The figure shows three views and two pictorial views of one solid part (mm, origin at its lowest corner). Answer the questions. A direction names the side the tool comes from. Round coordinates to 2 decimals unless told otherwise and drop trailing zeros. Write each loop counter-clockwise with the first axis right and the second up, starting at its lowest first coordinate (ties: lowest second). Pieces come first, ordered by that corner, then holes. Notation, with made-up numbers: M 15.25,68.5 L 63.25,68.5 A25 cw 63.25,83.5 Z; hole C 5,-36.75 d8. An arc over 180 degrees is marked long. One line per item, written item: value. Start each with the question number.
Q1. Given pin 1 Ø2 at (x, y) = (30.5, 20.5) entering from +Z, flat-ended and moving along its own axis, determine where the tip first touches the part or whether it passes through.
Q2. A tool of negligible diameter and unlimited length cuts with its end or side. For the marked faces 1 and 2, from which of +Z, -Z, +X, -X, +Y, -Y can it reach the whole face along a straight path? Write none if from no direction.
Q3. Find section D-D (x = 30). Write down the section's boundary in (y, z), and give its area (3 significant figures).
Q4. The mould has two halves that part along X. Classify the marked faces 3, 4 and 5: released by +X, released by -X, zero draft, split by the parting line, or undercut.
Q5. Find section C-C (z = 15.5). Write down the section's boundary in (x, y).
Q6. Find section B-B (x = 19). Write down the section's boundary in (y, z), and give its area (3 significant figures).
Q7. Consider probe 1 along Y at (x, z) = (17, 13.5); probe 2 along Y at (x, z) = (4, 14); probe 3 along Y at (x, z) = (15, 13). Determine where each line is inside the solid, lowest interval first.
Q8. Find section A-A (y = 5). Write down the section's boundary in (x, z), and give its area (3 significant figures).
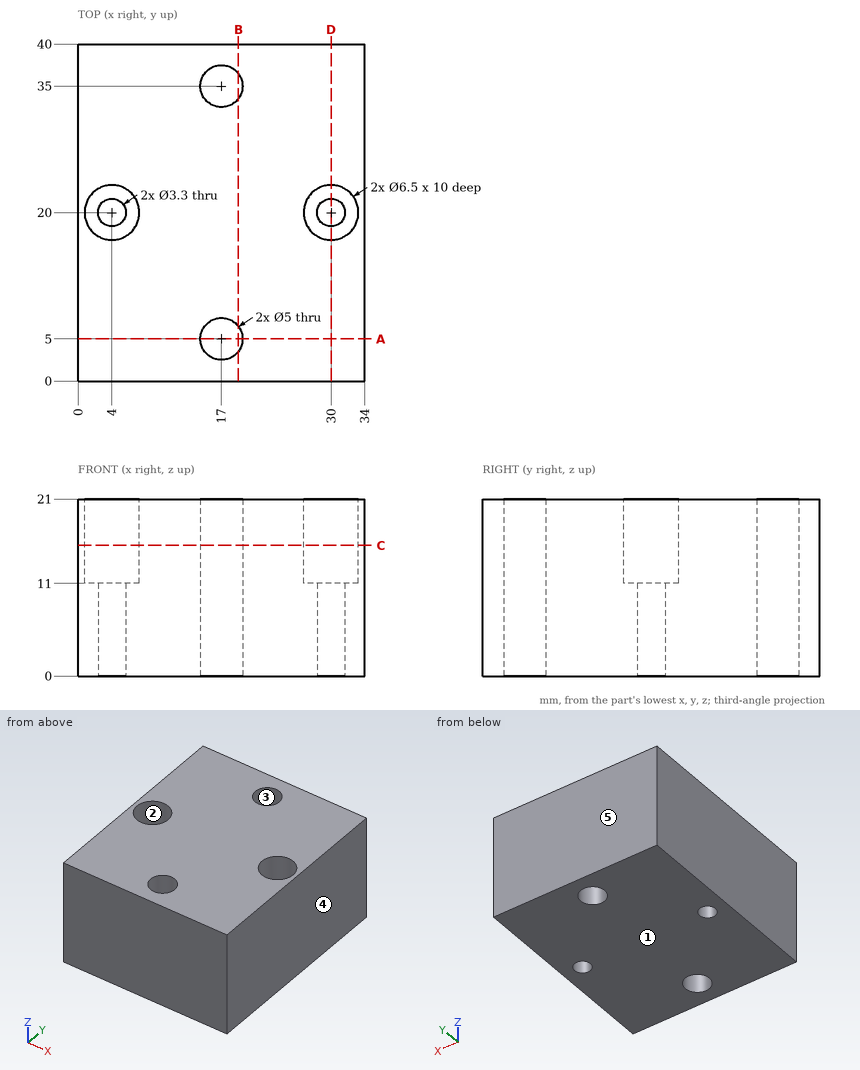
The answers:
1. pin 1: z = 11
2. face 1: -Z, +X, -X, +Y, -Y
2. face 2: +Z
3. outline: M 0,0 L 18.35,0 L 18.35,11 L 16.75,11 L 16.75,21 L 0,21 Z; M 21.65,0 L 40,0 L 40,21 L 23.25,21 L 23.25,11 L 21.65,11 Z
3. area: 739 mm2
4. face 3: undercut
4. face 4: released by +X
4. face 5: zero draft
5. outline: M 0,0 L 34,0 L 34,40 L 0,40 Z; hole C 4,20 d6.5; hole C 17,5 d5; hole C 17,35 d5; hole C 30,20 d6.5
6. outline: M 0,0 L 3.5,0 L 3.5,21 L 0,21 Z; M 6.5,0 L 33.5,0 L 33.5,21 L 6.5,21 Z; M 36.5,0 L 40,0 L 40,21 L 36.5,21 Z
6. area: 714 mm2
7. probe 1: 0 to 2.5, 7.5 to 32.5, 37.5 to 40
7. probe 2: 0 to 16.75, 23.25 to 40
7. probe 3: 0 to 3.5, 6.5 to 33.5, 36.5 to 40
8. outline: M 0,0 L 14.5,0 L 14.5,21 L 0,21 Z; M 19.5,0 L 34,0 L 34,21 L 19.5,21 Z
8. area: 609 mm2
